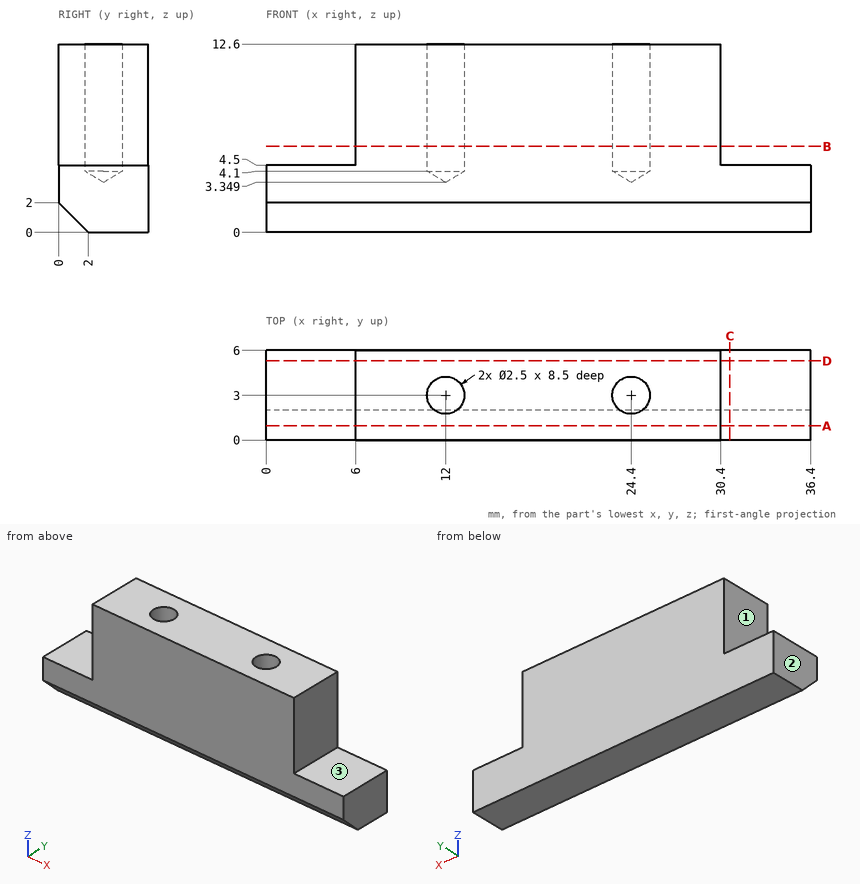
Geometry check sheet. Reference: drawing and pictorial views, mm from the part's lowest x, y, z. A direction names the side the tool comes from. Coordinates: 2 decimals unless noted, no trailing zeros. Write each loop counter-clockwise with the first axis right and the second up, starting at its lowest first coordinate (ties: lowest second). Pieces come first, ordered by that corner, then holes. Notation, with made-up numbers: (-19.75, 16) - (-6.75, 16) arc R30 ccw to (-6.75, 55) - close; hole circle Ø10 at (-33.5, -8). An arc over 180 degrees is marked (long way). One line per question, with ' | ' between items. Start each with the question number.
1. Section check C-C (x = 31). Enter the section's corners in (y, z).
2. Section check D-D (y = 5.3). Enter the section's corners in (x, z), plus the area to 3 significant figures.
3. Access from +Z, -Z, +X, -X, +Y, -Y to the whole of each face (thin tool, end or side, straight path). Record for the marked faces 1, 2 and 3.
4. Section check B-B (z = 5.75). Enter the section's corners in (x, y), plus the area to 3 significant figures.
5. Material ranges on line 1 along X through (y, z) = (3, 9.75); line 2 along Y through (x, z) = (24.4, 10.5); line 3 along X through (y, z) = (4.1, 10.25), recorded low to high.
6. Gauge pin test, flat end, axial feed: P1, Ø1.8, axis at x = 3, y = 3.5, coming from the +Z side. Record the tip position at first contact, or that the pin passes through.
7. Section check A-A (y = 0.95). Enter the section's corners in (x, z).
Computed values:
1) outline: (0, 2) - (2, 0) - (6, 0) - (6, 4.5) - (0, 4.5) - close
2) outline: (0, 0) - (36.4, 0) - (36.4, 4.5) - (30.4, 4.5) - (30.4, 12.6) - (6, 12.6) - (6, 4.5) - (0, 4.5) - close | area: 361 mm²
3) face 1: +Z, -X, +Y, -Y | face 2: +Z, -Z, -X, +Y, -Y | face 3: +Z, +X, +Y, -Y
4) outline: (6, 0) - (30.4, 0) - (30.4, 6) - (6, 6) - close; hole circle Ø2.5 at (12, 3); hole circle Ø2.5 at (24.4, 3) | area: 137 mm²
5) line 1: 6 to 10.75, 13.25 to 23.15, 25.65 to 30.4 | line 2: 0 to 1.75, 4.25 to 6 | line 3: 6 to 11.41, 12.59 to 23.81, 24.99 to 30.4
6) P1: z = 4.5
7) outline: (0, 1.05) - (36.4, 1.05) - (36.4, 4.5) - (30.4, 4.5) - (30.4, 12.6) - (6, 12.6) - (6, 4.5) - (0, 4.5) - close
